Input: dimensioned drawing with shaded views. Units: mm. Origin: part minimum x, y, z. A direction names the side the tool comes from. Coordinates: 2 decimals unless noted, no trailing zeros. Loops run counter-clockwise (first coordinate to the right, second up) from the corner with the lowest first, then second, coordinate; pieces in that order, holes last.
(1) Section D-D, the plane x = 2.5. Return loops of the section in (y, z).
(2) Line query: L1, parallel to Z at x = 8.5, y = 8.5; L2, parallel to Y at x = 2, z = 5.75; L3, parallel to Y at x = 4.25, z = 4.5. Output: solid intervals per line, ascending.
(3) Set-up query: the marked faces 1, 2, 3 and 4. Return all of +Z, -Z, +X, -X, +Y, -Y with unobstructed straight access to the full face (end or side cutting, diameter ignored); none if empty.
(4) Contact query for flat-ended pins moving along their axis: P1, Ø3.5, axis at x = 1.5, z = 6, coming from the +Y side; P2, Ø5, axis at x = 6, y = 4.5, coming from the +Z side; P3, Ø4, axis at y = 18.5, z = 5.5, coming from the -X side. Output: stop coordinate, or through.
(5) Section C-C, the plane y = 24.25. Return loops of the section in (x, z).
(6) Section A-A, the plane x = 11.5. Return loops of the section in (y, z).
(7) Section B-B, the plane z = 2. Return loops of the section in (x, y).
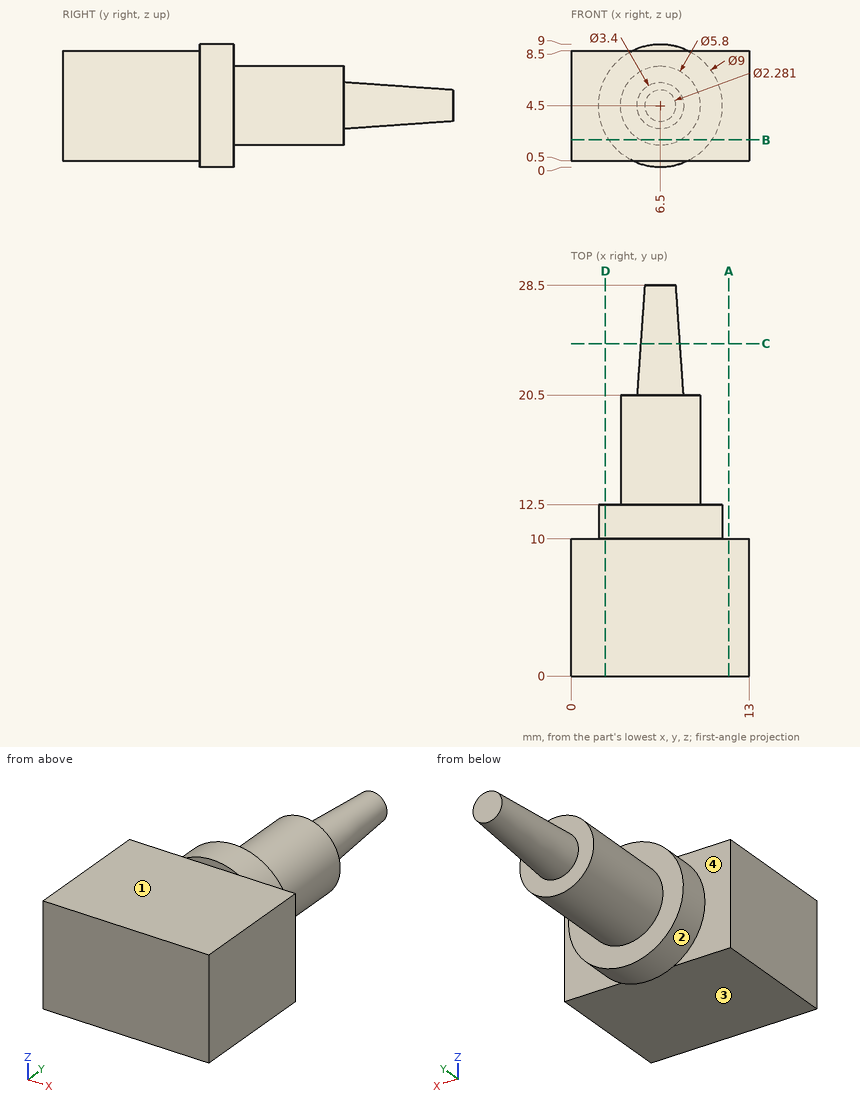
Report:
1. outline: (0, 0.5) - (10, 0.5) - (10, 2.44) - (12.5, 2.44) - (12.5, 6.56) - (10, 6.56) - (10, 8.5) - (0, 8.5) - close
2. L1: z = 0.5 to 8.5
2. L2: y = 0 to 10
2. L3: y = 0 to 20.5
3. face 1: +Z, +X, -X, -Y
3. face 2: +Y
3. face 3: -Z, +X, -X, -Y
3. face 4: -X, +Y
4. P1: stops at y = 12.5
4. P2: stops at z = 8.5
4. P3: stops at x = 3.6
5. outline: circle Ø2.88 at (6.5, 4.5)
6. outline: (0, 0.5) - (10, 0.5) - (10, 8.5) - (0, 8.5) - close
7. outline: (0, 0) - (13, 0) - (13, 10) - (10.24, 10) - (10.24, 12.5) - (7.97, 12.5) - (7.97, 20.5) - (5.03, 20.5) - (5.03, 12.5) - (2.76, 12.5) - (2.76, 10) - (0, 10) - close
